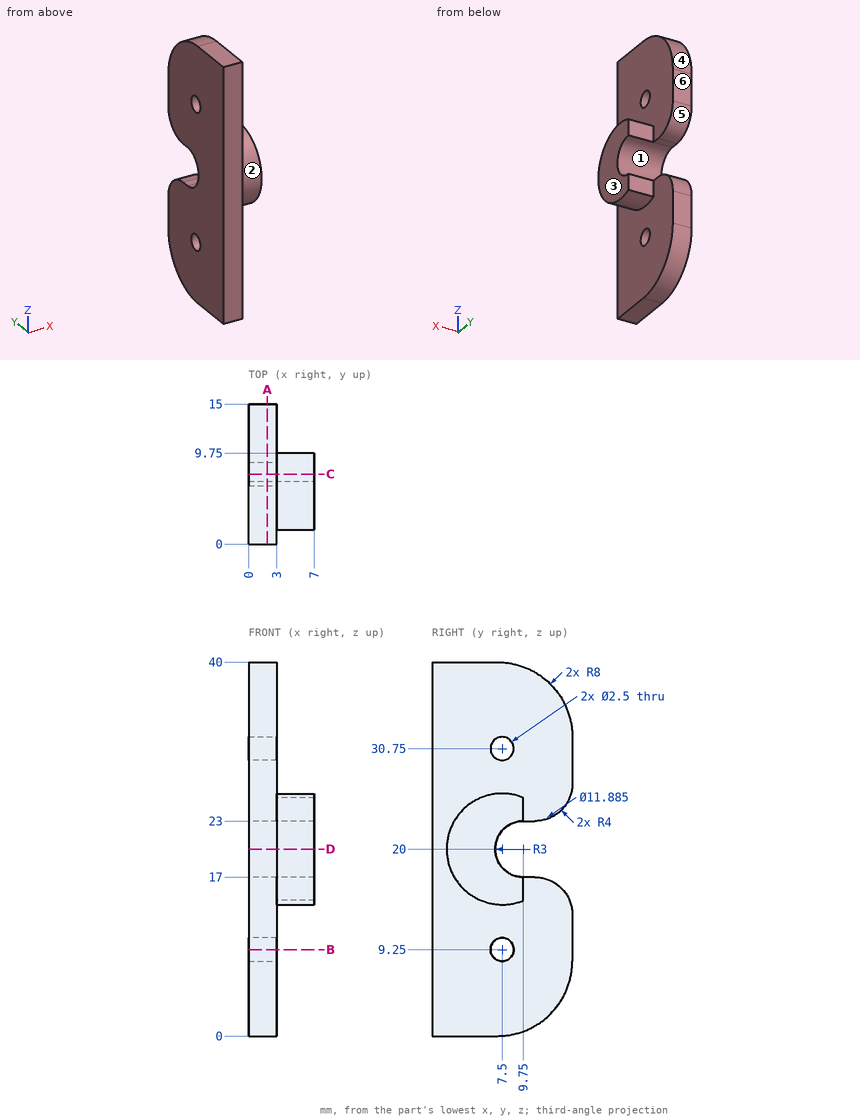
Here's the drawing with two shaded views (mm, measured from the low corner). I have some questions. A direction names the side the tool comes from. Coordinates: 2 decimals unless noted, no trailing zeros. Loops run counter-clockwise (first coordinate to the right, second up) from the corner with the lowest first, then second, coordinate; pieces in that order, holes last. Notation, with made-up numbers: (56, 9) -> (111, 9) arc R20 cw to (111, 31) -> close; hole circle Ø11 at (11, 5). An arc over 180 degrees is marked (long way). Use one line per item in the form item = value. Start each with the question number.
(1) If we section it at A-A (x = 2): Please give me the cut outline in (y, z).
(2) If we section it at D-D (z = 20): Please give me the cut outline in (x, y), then the cut area to 3 significant figures.
(3) If we section it at B-B (z = 9.25): Please give me the cut outline in (x, y).
(4) Will these pins go through, and if not, where does the flat tip stop? pin 1 (2 mm diameter, centred on x = 5, y = 12.5, fed in from -Z); pin 2 (8 mm diameter, centred on y = 13, z = 28.5, fed in from +X); pin 3 (1.4 mm diameter, centred on x = 1.5, y = 10.5, fed in from +Z); pin 4 (0.8 mm diameter, centred on x = 4.5, z = 15.5, fed in from +Y).
(5) Please list where these lines run through material, in increasing order: line 1 along Y through (x, z) = (1.55, 30.75); line 2 along X through (y, z) = (2.5, 25.5); line 3 along Z through (x, y) = (6.25, 8.25) (1 decimal).
(6) On a 3-axis mill with a long thin cutter (end or side, diameter ignored), from which of +Z, -Z, +X, -X, +Y, -Y can I reach the whole of each face in a straight line? I mean the marked faces 5 and 6. Say none if no direction works.
(7) If we section it at C-C (y = 7.5): Please give me the cut outline in (x, z).
(8) We'd pull the mould along Z, two halves only. Please class the marked faces 1, 2, 3 and 4: pulls with the +Z half, pulls with the -Z half, needs draft (parallel to the pull), parting line crosses it, or undercut.
Verdict:
q1.outline = (0, 0) -> (7, 0) arc R8 ccw to (15, 8) -> (15, 13) arc R4 ccw to (11, 17) -> (9.75, 17) arc R3 cw to (9.75, 23) -> (11, 23) arc R4 ccw to (15, 27) -> (15, 32) arc R8 ccw to (7, 40) -> (0, 40) -> close; hole circle Ø2.5 at (7.5, 9.25); hole circle Ø2.5 at (7.5, 30.75)
q2.outline = (0, 0) -> (3, 0) -> (3, 1.56) -> (7, 1.56) -> (7, 6.75) -> (0, 6.75) -> close
q2.area = 41.0 mm²
q3.outline = (0, 0) -> (3, 0) -> (3, 6.25) -> (0, 6.25) -> close; (0, 8.75) -> (3, 8.75) -> (3, 15) -> (0, 15) -> close
q4.pin_1 = through
q4.pin_2 = 3
q4.pin_3 = 39.49
q4.pin_4 = 9.75
q5.line_1 = 0 to 6.25, 8.75 to 15
q5.line_2 = 0 to 3
q5.line_3 = 14.1 to 17.4, 22.6 to 25.9
q6.face_5 = +X, -X, +Y
q6.face_6 = +Z, -Z, +X, -X, +Y
q7.outline = (0, 0.02) -> (3, 0.02) -> (3, 8) -> (0, 8) -> close; (0, 10.5) -> (3, 10.5) -> (3, 14.06) -> (7, 14.06) -> (7, 18.02) -> (0, 18.02) -> close; (0, 21.98) -> (7, 21.98) -> (7, 25.94) -> (3, 25.94) -> (3, 29.5) -> (0, 29.5) -> close; (0, 32) -> (3, 32) -> (3, 39.98) -> (0, 39.98) -> close
q8.face_1 = undercut
q8.face_2 = parting line crosses it
q8.face_3 = needs draft
q8.face_4 = pulls with the +Z half
